```python
from build123d import *

# Parameters (mm, degrees)
SKETCH1_R           = 13
BOSS_EXTRUDE1_DEPTH = 5
SKETCH12_R          = 4
CUT_EXTRUDE6_DEPTH  = 5
SKETCH13_R          = 6
BOSS_EXTRUDE7_DEPTH = 0.5
CUT_EXTRUDE7_START  = -0.5
SKETCH14_R          = 4
CUT_EXTRUDE7_DEPTH  = 0.5
BOSS_EXTRUDE8_DEPTH = 3
BOSS_EXTRUDE9_START = 30
SKETCH16_R          = 4
BOSS_EXTRUDE9_DEPTH = 30


with BuildPart() as part:
    # Sketch1 → Boss-Extrude1 (new body)
    with BuildSketch(Plane.XY):
        Circle(SKETCH1_R)
    extrude(amount=BOSS_EXTRUDE1_DEPTH)

    # Sketch12 → Cut-Extrude6 (cut)
    with BuildSketch(Plane.XY.offset(5)):
        Circle(SKETCH12_R)
    extrude(amount=-CUT_EXTRUDE6_DEPTH, mode=Mode.SUBTRACT)

    # Sketch13 → Boss-Extrude7 (add)
    with BuildSketch(Plane(origin=(0, 0, 0), x_dir=(-1, 0, 0), z_dir=(0, 0, -1))):
        with Locations(Location((0, 0, 0), (0, 0, 180))):
            Circle(SKETCH13_R)
    boss_extrude7 = extrude(amount=BOSS_EXTRUDE7_DEPTH)

    # Sketch14 → Cut-Extrude7 (cut)
    with BuildSketch(Plane(origin=(0, 0, -0.5), x_dir=(-1, 0, 0), z_dir=(0, 0, -1)).offset(CUT_EXTRUDE7_START)):
        with Locations(Location((0, 0, 0), (0, 0, 180))):
            Circle(SKETCH14_R)
    cut_extrude7 = extrude(amount=CUT_EXTRUDE7_DEPTH, mode=Mode.SUBTRACT)

    # Mirror2: Boss-Extrude7, Cut-Extrude7 across plane
    add(boss_extrude7.mirror(Plane(origin=(0, 0, 2.5), x_dir=(1, 0, 0), z_dir=(0, 0, -1))))
    add(cut_extrude7.mirror(Plane(origin=(0, 0, 2.5), x_dir=(1, 0, 0), z_dir=(0, 0, -1))), mode=Mode.SUBTRACT)

    # Sketch15 → Boss-Extrude8 (add)
    with BuildSketch(Plane(origin=(0, 0, -0.5), x_dir=(-1, 0, 0), z_dir=(0, 0, -1))):
        Polygon((5.743830787, 4.094007051), (-0.673598715, 7.021306902), (-6.417429503, 2.927299852), (-5.743830787, -4.094007051), (0.673598715, -7.021306902), (6.417429503, -2.927299852), align=None)
    extrude(amount=BOSS_EXTRUDE8_DEPTH)

    # Sketch16 → Boss-Extrude9 (add)
    with BuildSketch(Plane.XY.offset(-0.5).offset(BOSS_EXTRUDE9_START)):
        Circle(SKETCH16_R)
    extrude(amount=-BOSS_EXTRUDE9_DEPTH)


solid = part.part
```
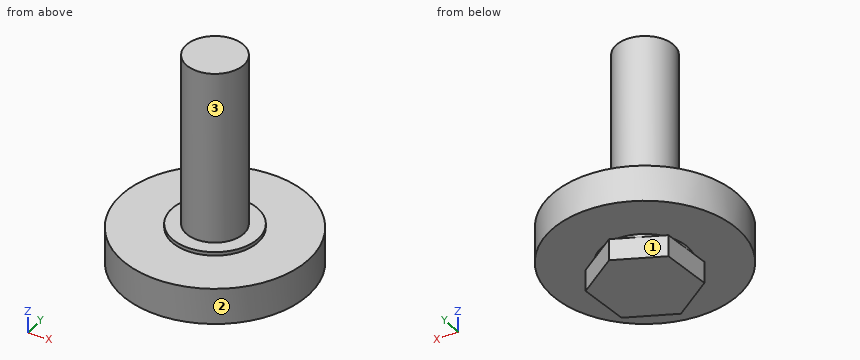
Work out the finished part from the listing and answer in its coordinate system (mm). Face numbers are marked on the shaded views. A direction names the side the tool comes from. Give positions to 0.01 mm unless a question says otherwise; leave off trailing zeros. Loops run counter-clockwise (first coordinate to the right, second up) from the corner with the lowest first, then second, coordinate; pieces in that order, holes last. Notation, with made-up numbers: (78, -17.5) -> (84, -17.5) arc R26 ccw to (84, 0.5) -> close; hole circle Ø5 at (55, 23.25). An arc over 180 degrees is marked (long way). Use CSV: the item, a comma, the result in double quotes.
1. Flat-ended cylindrical pins translate along their axes: pin 1 Ø12 at (x, z) = (7, 6.5) entering from +Y; pin 2 Ø12 at (x, z) = (-8, 6.5) entering from -Y; pin 3 Ø5 at (x, y) = (9.5, -8.5) entering from -Z. Find the tip coordinate at first contact, or state that the pin passes through.
Found:
pin 1,"y = 12.95"
pin 2,"y = -12.81"
pin 3,"z = 0"
2. The part is cut by section A-A (x = 0). Write down the section's boundary in (y, z).
Found:
outline,"(-13, 0) -> (-6, 0) -> (-6, -0.5) -> (-6.71, -0.5) -> (-6.71, -3.5) -> (6.71, -3.5) -> (6.71, -0.5) -> (6, -0.5) -> (6, 0) -> (13, 0) -> (13, 5) -> (6, 5) -> (6, 5.5) -> (4, 5.5) -> (4, 29.5) -> (-4, 29.5) -> (-4, 5.5) -> (-6, 5.5) -> (-6, 5) -> (-13, 5) -> close"
3. The part is cut by section B-B (z = 6). Write down the section's boundary in (x, y), then the cut area to 3 significant figures.
Found:
outline,"circle Ø8 at (0, 0)"
area,"50.3 mm^2"
4. The part is cut by section C-C (y = 0). Write down the section's boundary in (x, z), then the cut area to 3 significant figures.
Found:
outline,"(-13, 0) -> (-6, 0) -> (-6, -0.5) -> (-6.14, -0.5) -> (-6.14, -3.5) -> (6.14, -3.5) -> (6.14, -0.5) -> (6, -0.5) -> (6, 0) -> (13, 0) -> (13, 5) -> (6, 5) -> (6, 5.5) -> (4, 5.5) -> (4, 29.5) -> (-4, 29.5) -> (-4, 5.5) -> (-6, 5.5) -> (-6, 5) -> (-13, 5) -> close"
area,"371 mm^2"
5. The part is cut by section D-D (y = 5.5). Write down the section's boundary in (x, z).
Found:
outline,"(-11.78, 0) -> (-2.4, 0) -> (-2.4, -0.5) -> (-2.66, -0.5) -> (-2.66, -3.5) -> (2.81, -3.5) -> (2.81, -0.5) -> (2.4, -0.5) -> (2.4, 0) -> (11.78, 0) -> (11.78, 5) -> (2.4, 5) -> (2.4, 5.5) -> (-2.4, 5.5) -> (-2.4, 5) -> (-11.78, 5) -> close"
6. A tool of negligible diameter and unlimited length cuts with its end or side. For the marked faces 1, 2 and 3, from which of +Z, -Z, +X, -X, +Y, -Y can it reach the whole face along a straight path? Write none if from no direction.
Found:
face 1,"-Z, -X, +Y"
face 2,"+Z, -Z"
face 3,"+Z"
7. Straight lines are drawn through the part: line 1 (Z direction, x = 8.25, y = -5); line 2 (Y direction, x = 1.5, z = 25); line 3 (X direction, y = 2.25, z = 7.5). For each, find the intervals that lie inside material, in ascending order.
Found:
line 1,"0 to 5"
line 2,"-3.71 to 3.71"
line 3,"-3.31 to 3.31"
